Can you work these out from the drawing? Everything is in mm from the part's minimum corner. Round coordinates to 2 decimals unless told otherwise and drop trailing zeros. Write each loop counter-clockwise with the first axis right and the second up, starting at its lowest first coordinate (ties: lowest second). Pieces come first, ordered by that corner, then holes. Notation, with made-up numbers: (-33, 6.5) -> (-23, 6.5) arc R31 cw to (-23, 30.5) -> close; hole circle Ø1 at (76, 14.25). An arc over 180 degrees is marked (long way). Write item = value, one per line. Start each with the question number.
1) If I drill on line 1 (Y direction, x = 22, z = 1); line 2 (Y direction, x = 22, z = 6.5); line 3 (X direction, y = 20, z = 4.75) (1 decimal), over which ranges is the centre line in solid material (lowest first)?
2) Thinking about a two-plate mould opening in Y: for the marked faces 1, 2 and 3, which applies, +Y half, -Y half, draft (parallel to the pull), parting line (faces both ways), or undercut?
3) Imagine slicing it at C-C, the plane z = 5.75. Please give me the cut outline in (x, y), then the cut area to 3 significant figures.
4) Imagine slicing it at A-A, the plane y = 22. Please give me the cut outline in (x, z), then the cut area to 3 significant figures.
5) Imagine slicing it at D-D, the plane y = 12.75. Please give me the cut outline in (x, z).
6) I'm going to push flat-ended pins straight in: pin 1 (1 mm diameter, centred on x = 37.5, z = 4, fed in from -Y) (1 decimal); pin 2 (1.5 mm diameter, centred on x = 16, y = 14, fed in from -Z); pin 3 (1.5 mm diameter, centred on x = 38.5, y = 12.5, fed in from +Z); pin 4 (1 mm diameter, centred on y = 6, z = 4, fed in from +X). Where does each tip first touch, or does it pass through?
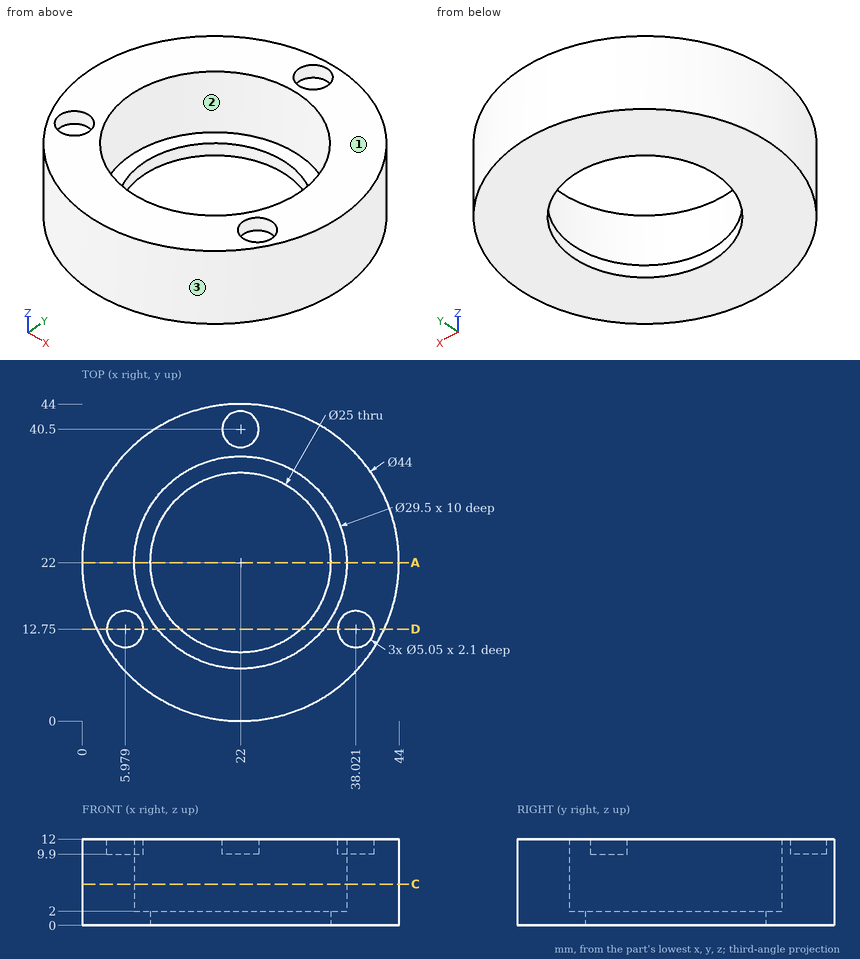
Reported:
q1.line_1 = 0 to 9.5, 34.5 to 44
q1.line_2 = 0 to 7.25, 36.75 to 44
q1.line_3 = 0.1 to 7.4, 36.6 to 43.9
q2.face_1 = draft
q2.face_2 = undercut
q2.face_3 = parting line
q3.outline = circle Ø44 at (22, 22); hole circle Ø29.5 at (22, 22)
q3.area = 837 mm²
q4.outline = (0, 0) -> (9.5, 0) -> (9.5, 2) -> (7.25, 2) -> (7.25, 12) -> (0, 12) -> close; (34.5, 0) -> (44, 0) -> (44, 12) -> (36.75, 12) -> (36.75, 2) -> (34.5, 2) -> close
q4.area = 183 mm²
q5.outline = (2.04, 0) -> (13.59, 0) -> (13.59, 2) -> (10.51, 2) -> (10.51, 12) -> (8.5, 12) -> (8.5, 9.9) -> (3.45, 9.9) -> (3.45, 12) -> (2.04, 12) -> close; (30.41, 0) -> (41.96, 0) -> (41.96, 12) -> (40.55, 12) -> (40.55, 9.9) -> (35.5, 9.9) -> (35.5, 12) -> (33.49, 12) -> (33.49, 2) -> (30.41, 2) -> close
q6.pin_1 = 5.9
q6.pin_2 = through
q6.pin_3 = 9.9
q6.pin_4 = 37.61
